Here's how the part is built. I have some questions about the finished solid (model axes, mm). A direction names the side the tool comes from. Give positions to 0.01 mm unless a question says otherwise; leave off trailing zeros. Loops run counter-clockwise (first coordinate to the right, second up) from the corner with the lowest first, then second, coordinate; pieces in that order, holes last.
Q1. If we section it at C-C (x = 0): Please give me the cut outline in (y, z), plus the area to 4 significant figures.
Q2. We'd pull the mould along Y, two halves only. Please class faces 3 (the face through (-7.4, -0.9, 10)), 4 (the face through (0.289, -9.245, 3.819)), 5 (the face through (-0.227, -7.246, 3.819)): +Y half, -Y half, draft (parallel to the pull), parting line (faces both ways), or undercut.
Q3. If we section it at A-A (y = 0): Please give me the cut outline in (x, z), plus the area to 3 significant figures.
Q4. I need wall thicknesses on line 1 (X direction, y = 0, z = 2); line 2 (X direction, y = -1.75, z = 6.5); line 3 (Y direction, x = -6.25, z = 8.25). Which ranges of each line are inside material? Lowest first, please.
Q5. If we section it at B-B (x = 6.75): Please give me the cut outline in (y, z).
Q6. Will these pins go through, and if not, where does the flat tip stop? P1, Ø1, axis at x = -3, z = 6.5, coming from the -Y side; P2, Ø2, axis at x = -3.5, z = 8, coming from the +Y side; P3, Ø1, axis at x = 3.5, z = 8, coming from the +Y side.
Q7. If we section it at D-D (x = -5): Please give me the cut outline in (y, z).
Q8. For faces 1 (the face through (7.4, -0.9, 10)), 2 (the face through (-0.1, -7.4, 5)), which set-ups out of +Z, -Z, +X, -X, +Y, -Y let a thin tool reach every point of the face, with its end or its side?
from build123d import *

# Parameters (mm, degrees)
EXTRUDE_569_DEPTH           = 10
CUT_EXTRUDE_2098_DEPTH      = 21.508286309
CUT_EXTRUDE_2098_DEPTH_BACK = 21.508286309
SKETCH_6_R                  = 4.5


with BuildPart() as part:
    # Эскиз1 → Extrude 569 (new body)
    with BuildSketch(Plane.XY):
        with BuildLine():
            ThreePointArc((-5.712121212, 4.464770012), (0, -7.25), (5.712121212, 4.464770012))
            ThreePointArc((5.712121212, 4.464770012), (5.884169654, 5.868479146), (7.287878788, 5.696430705))
            ThreePointArc((7.287878788, 5.696430705), (0, -9.25), (-7.287878788, 5.696430705))
            ThreePointArc((-7.287878788, 5.696430705), (-5.884169654, 5.868479146), (-5.712121212, 4.464770012))
        make_face()
    extrude(amount=EXTRUDE_569_DEPTH)

    # Эскиз6 → Cut-Extrude 2098 (cut, two sides: drawn at the far end of the back side and taken through both)
    with BuildSketch(Plane(origin=(0, -9.25, 0), x_dir=(-1, 0, 0), z_dir=(0, -1, 0)).offset(-CUT_EXTRUDE_2098_DEPTH_BACK)):
        with Locations((0, -9.5)):
            Circle(SKETCH_6_R)
    extrude(amount=CUT_EXTRUDE_2098_DEPTH + CUT_EXTRUDE_2098_DEPTH_BACK, mode=Mode.SUBTRACT)


solid = part.part
Check sheet entries:
1. outline: (-9.25, 0) - (-7.25, 0) - (-7.25, 5) - (-9.25, 5) - close
1. area: 10.00 mm2
2. face 3: draft
2. face 4: parting line
2. face 5: undercut
3. outline: (-9.25, 0) - (-7.25, 0) - (-7.25, 10) - (-9.25, 10) - close; (7.25, 0) - (9.25, 0) - (9.25, 10) - (7.25, 10) - close
3. area: 40.0 mm2
4. line 1: x = -9.25 to -7.25, 7.25 to 9.25
4. line 2: x = -9.08 to -7.04, 7.04 to 9.08
4. line 3: y = -6.82 to -3.67, 3.67 to 6.05
5. outline: (-6.32, 0) - (-2.65, 0) - (-2.65, 10) - (-6.32, 10) - close; (2.65, 0) - (6.05, 0) - (6.05, 10) - (2.65, 10) - close
6. P1: stops at y = -8.8
6. P2: stops at y = -5.68
6. P3: passes through
7. outline: (-7.78, 0) - (-5.25, 0) - (-5.25, 10) - (-7.78, 10) - close
8. face 1: +Z, +X, -X, +Y, -Y
8. face 2: +Y, -Y
